from build123d import *

# Parameters (mm, degrees)
SKETCH1_R           = 15
BOSS_EXTRUDE1_DEPTH = 20
SKETCH2_R           = 10
BOSS_EXTRUDE2_DEPTH = 2000
SKETCH3_R           = 10
BOSS_EXTRUDE3_DEPTH = 50


with BuildPart() as part:
    # Sketch1 → Boss-Extrude1 (new body)
    with BuildSketch(Plane(origin=(0, 0, 0), x_dir=(1, 0, 0), z_dir=(0, 1, 0))):
        Circle(SKETCH1_R)
    extrude(amount=BOSS_EXTRUDE1_DEPTH)

    # Sketch2 → Boss-Extrude2 (add)
    with BuildSketch(Plane(origin=(0, 0, 0), x_dir=(0, 0, -1), z_dir=(1, 0, 0))):
        with Locations((0, 10)):
            Circle(SKETCH2_R)
    extrude(amount=BOSS_EXTRUDE2_DEPTH)

    # Sketch3 → Boss-Extrude3 (add)
    with BuildSketch(Plane(origin=(0, 0, 0), x_dir=(1, 0, 0), z_dir=(0, 1, 0))):
        with Locations((2000, 0)):
            Circle(SKETCH3_R)
    extrude(amount=BOSS_EXTRUDE3_DEPTH)


solid = part.part
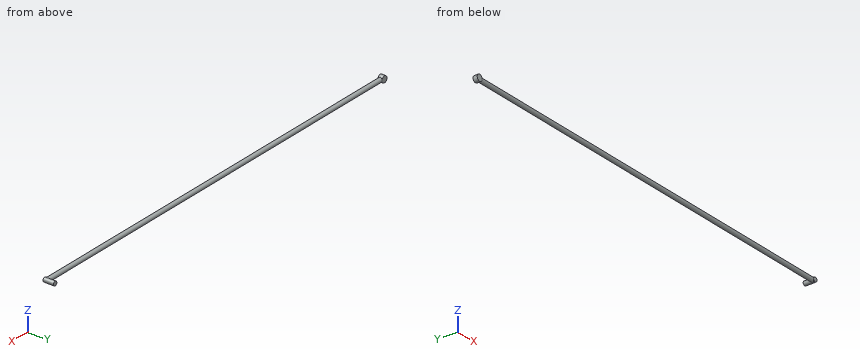
The listing builds one solid part. Answer for the finished solid, in the listing's coordinates (mm). Give positions to 0.01 mm unless a question says otherwise; leave off trailing zeros. Write each loop counter-clockwise with the first axis right and the second up, starting at its lowest first coordinate (ties: lowest second). Pieces come first, ordered by that corner, then holes. Notation, with made-up numbers: (-10, 45.5) -> (-3, 45.5) arc R25 ccw to (-3, 57.5) -> close; hole circle Ø7 at (9.5, 76). An arc over 180 degrees is marked (long way). One line per question, with ' | ' between items. Start each with the question number.
1. Given pin 1 Ø4 at (x, y) = (1002, 17) entering from -Z; pin 2 Ø1.5 at (x, y) = (1181.5, 6.5) entering from +Z; pin 3 Ø1.5 at (y, z) = (17, -6.5) entering from +X; pin 4 Ø5 at (x, y) = (1724, 24) entering from +Z, each flat-ended and moving along its own axis, determine where each tip first touches the part or whether it passes through.
2. Find the intervals of material crossed by probe 1 along Y at (x, z) = (1337, 1.5); probe 2 along X at (y, z) = (26.5, 1.5); probe 3 along Z at (x, y) = (497.5, 10.5), in increasing order.
3. Section A-A (y = 10) is taken. Determine the outline of the cut face in (x, z), plus the area to 3 significant figures.
4. Section B-B (x = 1690) is taken. Determine the outline of the cut face in (y, z), plus the area to 3 significant figures.
Response values:
1) pin 1: z = -8.66 | pin 2: z = 9.61 | pin 3: x = 2008.18 | pin 4: through
2) probe 1: 0.11 to 19.89 | probe 2: 1990.11 to 2009.89 | probe 3: -9.99 to 9.99
3) outline: (11.18, -10) -> (2000, -10) arc R10 ccw to (2000, 10) -> (11.18, 10) arc R15 ccw (long way) to start | area: 40,600 mm2
4) outline: circle Ø20 at (10, 0) | area: 314 mm2
